```python
from build123d import *

# Parameters (mm, degrees)
SKETCH1_W           = 50.8
SKETCH1_H           = 22.86
BOSS_EXTRUDE1_DEPTH = 3.175
FILLET1_R           = 10.16
SKETCH3_R           = 1.9685
CUT_EXTRUDE1_DEPTH  = 29.033649869
FILLET3_R           = 10.16
SCALE1_SCALE_X      = 0.84
SCALE1_SCALE_Y      = 1
SCALE1_SCALE_Z      = 0.84
CUT_EXTRUDE2_DEPTH  = 24.662282921
FILLET4_R           = 3.175
FILLET5_DEPTH       = 3.175


with BuildPart() as part:
    # Sketch1 → Boss-Extrude1 (new body)
    with BuildSketch(Plane(origin=(0, 0, 0), x_dir=(1, 0, 0), z_dir=(0, 1, 0))):
        Rectangle(SKETCH1_W, SKETCH1_H)
    extrude(amount=BOSS_EXTRUDE1_DEPTH)

    # Fillet1
    fillet1_edges = [part.edges().sort_by_distance(p)[0] for p in [
        (25.4, 1.5875, 11.43),
        (-25.4, 1.5875, 11.43),
    ]]
    fillet(fillet1_edges, radius=FILLET1_R)

    # Sketch3 → Cut-Extrude1 (cut, through all)
    with BuildSketch(Plane(origin=(0, 3.175, 0), x_dir=(1, 0, 0), z_dir=(0, 1, 0))):
        with Locations(Location((15.24, -1.27, 0), (0, 0, 270))):
            Circle(SKETCH3_R)
        with Locations(Location((16.637, 6.994763457, 0), (0, 0, 270))):
            Circle(SKETCH3_R)
        with Locations(Location((-3.81, -1.27, 0), (0, 0, 270))):
            Circle(SKETCH3_R)
    extrude(amount=-CUT_EXTRUDE1_DEPTH, mode=Mode.SUBTRACT)

    # Fillet3
    fillet3_edges = [part.edges().sort_by_distance(p)[0] for p in [
        (-25.4, 1.5875, -11.43),
        (25.4, 1.5875, -11.43),
    ]]
    fillet(fillet3_edges, radius=FILLET3_R)


with BuildPart() as part_1:
    # Scale1: scaled about (-0.329754669, 1.5875, 0.052338299)
    add(part.part.scale((SCALE1_SCALE_X, SCALE1_SCALE_Y, SCALE1_SCALE_Z), about=(-0.329754669, 1.5875, 0.052338299)))

    # Sketch4 → Cut-Extrude2 (cut, through all)
    with BuildSketch(Plane(origin=(0, 3.175, 0), x_dir=(1, 0, 0), z_dir=(0, 1, 0))):
        with BuildLine():
            Line((12.984828754, -7.325177491), (12.984828754, -9.609574128))
            Line((12.984828754, -9.609574128), (-21.388760747, -9.609574128))
            Line((-21.388760747, -9.609574128), (-21.388760747, 9.592825872))
            Line((-21.388760747, 9.592825872), (6.353119253, 9.592825872))
            Line((6.353119253, 9.592825872), (6.353119253, 7.824824044))
            Line((6.353119253, 7.824824044), (12.984828754, 7.824824044))
            Line((12.984828754, 7.824824044), (12.984828754, 5.174822509))
            Line((12.984828754, 5.174822509), (12.384828754, 5.174822509))
            ThreePointArc((12.384828754, 5.174822509), (8.374442055, 3.924822509), (12.384828754, 2.674822509))
            Line((12.384828754, 2.674822509), (12.984828754, 2.674822509))
            Line((12.984828754, 2.674822509), (12.984828754, -4.825177491))
            Line((12.984828754, -4.825177491), (12.384828754, -4.825177491))
            ThreePointArc((12.384828754, -4.825177491), (8.374442055, -6.075177491), (12.384828754, -7.325177491))
            Line((12.384828754, -7.325177491), (12.984828754, -7.325177491))
        make_face()
    extrude(amount=-CUT_EXTRUDE2_DEPTH, mode=Mode.SUBTRACT)

    # Fillet4
    # the kernel refuses this fillet: 3.175 mm, written as the material it takes off along each edge
    with BuildSketch(Plane(origin=(6.353119253, 10.290555646, -9.592825872), x_dir=(1.0, 0, -2.4331567057805564e-11), z_dir=(0, -1, 0))) as fillet4_piece_1:
        with BuildLine():
            CenterArc((2.846222258, 3.175), FILLET4_R, 206.304974961, 63.695025041)
            Line((0, 1.768001828), (-0.056924445, 1.739861865))
            ThreePointArc((-0.056924445, 1.739861865), (-0.0635, 0.884000914), (-0.0635, 0))
            Line((-0.0635, 0), (0, -0.0635))
            Line((0, -0.0635), (2.846222258, -0.0635))
            Line((2.846222258, -0.0635), (2.846222258, 0))
        make_face()
    extrude(amount=17.406111292, mode=Mode.SUBTRACT)

    # Fillet5: read off the stored shape, not the designer's step
    # Fillet5 outline → Fillet5 (add)
    with BuildSketch(Plane(origin=(0, 0, 0), x_dir=(1, 0, 0), z_dir=(0, 1, 0))):
        with BuildLine():
            ThreePointArc((12.351058447, 7.824824044), (12.785881926, 7.65259131), (12.984828754, 7.22932339))
            Line((12.984828754, 7.22932339), (12.984828754, 7.824824044))
            Line((12.984828754, 7.824824044), (12.351058447, 7.824824044))
        make_face()
    extrude(amount=FILLET5_DEPTH)


solid = part_1.part
```
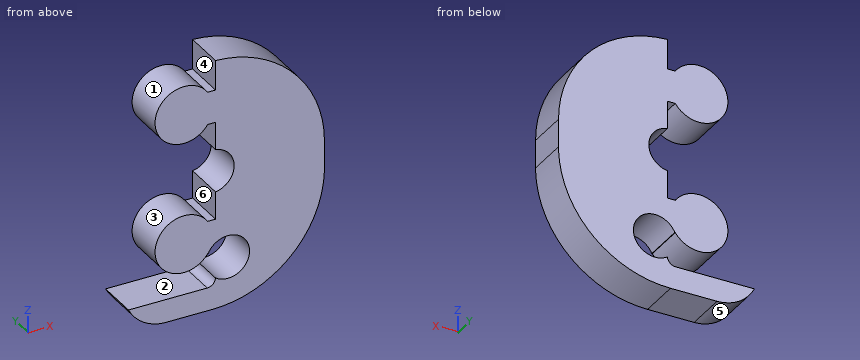
Read the model definition and answer for the solid it produces. Units are mm, in the model's axes. Face numbers are marked on the shaded views. A direction names the side the tool comes from. Give positions to 0.01 mm unless a question says otherwise; leave off trailing zeros. Answer as a JSON object with one key per item and string values.
1) A tool of negligible diameter and unlimited length cuts with its end or side. For the marked faces 1 and 2, from which of +Z, -Z, +X, -X, +Y, -Y can it reach the whole face along a straight path? Write none if from no direction.
Findings below:
{"face 1": "+Y, -Y", "face 2": "-X, +Y, -Y"}
2) Flat-ended cylindrical pins translate along their axes: pin 1 Ø0.6 at (y, z) = (2, 3.5) entering from -X; pin 2 Ø1 at (x, y) = (10, 2.5) entering from +Z; pin 3 Ø1.5 at (x, y) = (14, 3) entering from +Z. Find the tip coordinate at first contact, or state that the pin passes through.
Findings below:
{"pin 1": "stops at x = 12.98", "pin 2": "stops at z = 8.27", "pin 3": "stops at z = 9.59"}
3) Section A-A on x = 9.5 is taken. Count the separate pieces of the cut face and the enclosed holes in it, then the cut area to 3 significant figures.
Findings below:
{"separate pieces": "3", "enclosed holes": "0", "area": "30.0 mm^2"}
4) For a pull along Z with two mould halves and no side action, classify the marked faces 3, 4, 5 and 6 as pulls with the +Z half, pulls with the -Z half, needs draft (parallel to the pull), parting line crosses it, or undercut.
Findings below:
{"face 3": "undercut", "face 4": "needs draft", "face 5": "pulls with the -Z half", "face 6": "undercut"}
5) Straight lines are drawn through the part: probe 1 along Z at (x, y) = (10.5, 2.55); probe 2 along Z at (x, y) = (9.5, 2.7); probe 3 along X at (y, z) = (2.05, -4.75). For each, find the intervals that lie inside material, in ascending order. Write a range as from..to.
Findings below:
{"probe 1": "z = -9.59..-7.82, -6.12..-1.73, 3.88..8.27", "probe 2": "z = -9.59..-7.82, -5.84..-2.01, 4.16..7.99", "probe 3": "x = 8.54..12.7, 15.14..20.44"}
